from build123d import *

# Parameters (mm, degrees)
SKETCH1_W           = 2.1
SKETCH1_H           = 2.1
BOSS_EXTRUDE1_DEPTH = 1
SKETCH4_W           = 2.1
SKETCH4_H           = 2.1
BOSS_EXTRUDE3_DEPTH = 2
SWEEP4_START        = -1.05
SWEEP4_DEPTH        = 2.1
SKETCH7_W           = 2.1
SKETCH7_H           = 2.1
CUT_EXTRUDE1_DEPTH  = 2


# Read off the part's stored shape, not the designer's step: Sweep4
with BuildPart() as part:
    # Sketch1 → Boss-Extrude1 (new body)
    with BuildSketch(Plane.XY):
        Rectangle(SKETCH1_W, SKETCH1_H)
    extrude(amount=BOSS_EXTRUDE1_DEPTH)

    # Sketch4 → Boss-Extrude3 (add)
    with BuildSketch(Plane.XY):
        Rectangle(SKETCH4_W, SKETCH4_H)
    extrude(amount=-BOSS_EXTRUDE3_DEPTH)

    # Sweep4 outline → Sweep4 (add)
    with BuildSketch(Plane(origin=(0, 0, 0), x_dir=(1, 0, 0), z_dir=(0, 1, 0)).offset(SWEEP4_START)):
        with BuildLine():
            Line((7.04999865, 11.165148445), (7.04999919, 11.5))
            Line((7.04999919, 11.5), (4.94999919, 11.5))
            Line((4.94999919, 11.5), (4.94999865, 11.165148445))
            ThreePointArc((4.94999865, 11.165148445), (4.141466162, 8.453922768), (1.979999995, 6.628399977))
            ThreePointArc((1.979999995, 6.628399977), (-0.225133297, 4.765998667), (-1.05, 2))
            Line((-1.05, 2), (1.05, 2))
            ThreePointArc((1.05, 2), (1.531852827, 3.615781399), (2.819999682, 4.703719521))
            ThreePointArc((2.819999682, 4.703719521), (5.898452285, 7.303705501), (7.04999865, 11.165148445))
        make_face()
    sweep4 = extrude(amount=SWEEP4_DEPTH)

    # Mirror1: Sweep4 across plane
    add(sweep4.mirror(Plane(origin=(0, 0, 0), x_dir=(0, 0, 1), z_dir=(1, 0, 0))))

    # Sketch7 → Cut-Extrude1 (cut)
    with BuildSketch(Plane.XY.offset(1)):
        Rectangle(SKETCH7_W, SKETCH7_H)
    extrude(amount=-CUT_EXTRUDE1_DEPTH, mode=Mode.SUBTRACT)


solid = part.part
Read the model definition and answer for the solid it produces. Units are mm, in the model's axes. A direction names the side the tool comes from. Round coordinates to 2 decimals unless told otherwise and drop trailing zeros. Order: outer loops, then holes, each group sorted by start corner. A loop starts at its lowest first (then second) coordinate and runs counter-clockwise, first axis right, second up. Notation, with made-up numbers: (-14.5, -24.5) - (21.5, -24.5) arc R34 ccw to (21.5, 5.5) - close; hole circle Ø10 at (55, 57.5). An arc over 180 degrees is marked (long way). Use one line per item in the form item = value. Start each with the question number.
(1) The part is cut by section D-D (x = 0.5). Give the vertices of the cut face in (y, z).
(2) Find the intervals of material crossed by line 1 along X through (y, z) = (0.45, -7.25); line 2 along X through (y, z) = (-0.65, -9); line 3 along X through (y, z) = (0.95, -5), in increasing order. Write a range as from..to.
(3) Flat-ended cylindrical pins translate along their axes: pin 1 Ø6 at (x, z) = (2.5, -9) entering from -Y; pin 2 Ø0.5 at (y, z) = (0.5, -1.5) entering from +X; pin 3 Ø0.8 at (y, z) = (0.5, -1.5) entering from -X; pin 4 Ø1 at (x, y) = (-5, 0.5) entering from +Z. Find the tip coordinate at first contact, or state that the pin passes through.
(4) Determine the mould class of faces 1 (the face through (-5.87, -0.01, -7.26)), 2 (the face through (-4.163, -0.015, -8.488)), 3 (the face through (2, -1.05, -6)) for opening direction X: +X half, -X half, draft (parallel to the pull), parting line (faces both ways), or undercut.
(5) The part is cut by section C-C (z = -7.75). Give the vertices of the cut face in (x, y), then the cut area to 3 significant figures.
(6) The part is cut by section A-A (y = -0.55). Give the vertices of the cut face in (x, z).
(7) For faces 4 (the face through (-1.05, 0, -1.5)), 5 (the face through (4.163, -0.015, -8.488)), 6 (the face through (1.05, 0, -1.5)), 7 (the face through (0, 0, -1)), determine the directions among +Z, -Z, +X, -X, +Y, -Y from which every point of the face is accessible in a straight line to the end or side of a thin tool.
(8) The part is cut by section B-B (z = -10). Give the vertices of the cut face in (x, y).
Checked values:
q1.outline = (-1.05, -5.64) - (1.05, -5.64) - (1.05, -1) - (-1.05, -1) - close
q2.line_1 = -5.86..-3.03, 3.03..5.86
q2.line_2 = -6.71..-4.45, 4.45..6.71
q2.line_3 = -3.42..3.42
q3.pin_1 = -1.05
q3.pin_2 = 1.05
q3.pin_3 = -1.05
q3.pin_4 = -5.74
q4.face_1 = -X half
q4.face_2 = undercut
q4.face_3 = draft
q5.outline = (-6.17, -1.05) - (-3.58, -1.05) - (-3.58, 1.05) - (-6.17, 1.05) - close; (3.58, -1.05) - (6.17, -1.05) - (6.17, 1.05) - (3.58, 1.05) - close
q5.area = 10.9 mm^2
q6.outline = (-7.05, -11.5) - (-4.95, -11.5) - (-4.95, -11.17) arc R4.95 cw to (-1.98, -6.63) arc R5.05 ccw to (0, -5.08) arc R5.05 ccw to (1.98, -6.63) arc R4.95 cw to (4.95, -11.17) - (4.95, -11.5) - (7.05, -11.5) - (7.05, -11.17) arc R7.05 ccw to (2.82, -4.7) arc R2.95 cw to (1.05, -2) - (1.05, -1) - (-1.05, -1) - (-1.05, -2) arc R2.95 cw to (-2.82, -4.7) arc R7.05 ccw to (-7.05, -11.17) - close
q7.face_4 = +Z, -X, +Y, -Y
q7.face_5 = -Z, +Y, -Y
q7.face_6 = +Z, +X, +Y, -Y
q7.face_7 = +Z, +X, -X, +Y, -Y
q8.outline = (-6.95, -1.05) - (-4.81, -1.05) - (-4.81, 1.05) - (-6.95, 1.05) - close; (4.81, -1.05) - (6.95, -1.05) - (6.95, 1.05) - (4.81, 1.05) - close
